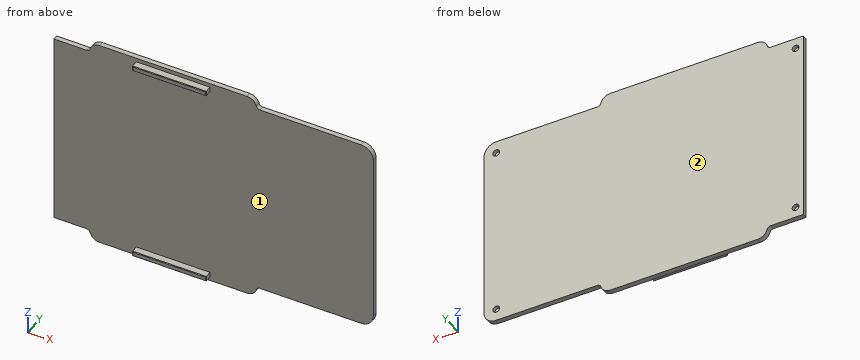
```python
from build123d import *

# Parameters (mm, degrees)
BOSS_EXTRUDE1_DEPTH = 4
FILLET1_R           = 3
FILLET2_R           = 8
FILLET3_R           = 10
SKETCH2_R           = 2.75
CUT_EXTRUDE2_DEPTH  = 4
SKETCH3_W           = 60
SKETCH3_H           = 4
BOSS_EXTRUDE2_DEPTH = 6
CHAMFER1_SIZE       = 0.5
SKETCH2_3_R         = 2.75
BOSS_EXTRUDE3_DEPTH = 1


with BuildPart() as part:
    # Sketch1 → Boss-Extrude1 (new body)
    with BuildSketch(Plane(origin=(0, 0, 0), x_dir=(1, 0, 0), z_dir=(0, 1, 0))):
        Polygon((29.5, 168.2), (29.5, 160), (0, 160), (0, 80), (0, 0), (29.5, 0), (29.5, -8.2), (164.72, -8.2), (164.72, 0), (260, 0), (260, 160), (164.72, 160), (164.72, 168.2), align=None)
    extrude(amount=BOSS_EXTRUDE1_DEPTH)

    # Fillet1
    fillet1_edges = [part.edges().sort_by_distance(p)[0] for p in [
        (164.72, 2, 0),
        (29.5, 2, 0),
        (29.5, 2, -160),
        (164.72, 2, -160),
    ]]
    fillet(fillet1_edges, radius=FILLET1_R)

    # Fillet2
    fillet2_edges = [part.edges().sort_by_distance(p)[0] for p in [
        (29.5, 2, -168.2),
        (164.72, 2, -168.2),
        (29.5, 2, 8.2),
        (164.72, 2, 8.2),
    ]]
    fillet(fillet2_edges, radius=FILLET2_R)

    # Fillet3
    fillet3_edges = [part.edges().sort_by_distance(p)[0] for p in [
        (260, 2, -160),
        (260, 2, 0),
    ]]
    fillet(fillet3_edges, radius=FILLET3_R)

    # Sketch2 → Cut-Extrude2 (cut)
    with BuildSketch(Plane(origin=(0, 0, 0), x_dir=(1, 0, 0), z_dir=(0, 1, 0))):
        with Locations((6.25, 151.25)):
            Circle(SKETCH2_R)
        with Locations((250, 150)):
            Circle(SKETCH2_R)
        with Locations((250, 10)):
            Circle(SKETCH2_R)
        with Locations((6.25, 8.75)):
            Circle(SKETCH2_R)
    extrude(amount=CUT_EXTRUDE2_DEPTH, mode=Mode.SUBTRACT)

    # Sketch3 → Boss-Extrude2 (add)
    with BuildSketch(Plane(origin=(0, 0, 0), x_dir=(1, 0, 0), z_dir=(0, 1, 0))):
        with Locations((97.11, 163)):
            Rectangle(SKETCH3_W, SKETCH3_H)
        with Locations((97.11, -3)):
            Rectangle(SKETCH3_W, SKETCH3_H)
    extrude(amount=-BOSS_EXTRUDE2_DEPTH)

    # Chamfer1
    chamfer1_edges = [part.edges().sort_by_distance(p)[0] for p in [
        (67.11, -6, -163),
        (97.11, -6, -161),
        (97.11, -6, -165),
        (127.11, -6, -163),
        (127.11, -6, 3),
        (97.11, -6, 5),
        (67.11, -6, 3),
        (97.11, -6, 1),
    ]]
    chamfer(chamfer1_edges, length=CHAMFER1_SIZE)

    # Sketch2<3> → Boss-Extrude3 (add)
    with BuildSketch(Plane(origin=(0, 0, 0), x_dir=(1, 0, 0), z_dir=(0, 1, 0))):
        with Locations((6.25, 151.25)):
            Circle(SKETCH2_3_R)
        with Locations((250, 150)):
            Circle(SKETCH2_3_R)
        with Locations((250, 10)):
            Circle(SKETCH2_3_R)
        with Locations((6.25, 8.75)):
            Circle(SKETCH2_3_R)
    extrude(amount=BOSS_EXTRUDE3_DEPTH)


solid = part.part
```
Design review of the part built by this model. Coordinates are the model's own, in mm. Face numbers are marked on the shaded views. Round coordinates to 2 decimals unless told otherwise and drop trailing zeros. Order: outer loops, then holes, each group sorted by start corner. A loop starts at its lowest first (then second) coordinate and runs counter-clockwise, first axis right, second up. Notation, with made-up numbers: (25, 19) - (55, 19) arc R30 ccw to (55, 44) - close; hole circle Ø8 at (53.25, 34). An arc over 180 degrees is marked (long way). Return JSON: item names as keys, results as strings.
Q1. Consider section C-C on z = -32. Write out the cut boundary in (x, y).
Computed values:
{"outline": "(0, 0) - (260, 0) - (260, 4) - (0, 4) - close"}
Q2. Consider section D-D on x = 122. Write out the cut boundary in (y, z), plus the area to 3 significant figures.
Computed values:
{"outline": "(-6, -164.5) - (-5.5, -165) - (0, -165) - (0, -168.2) - (4, -168.2) - (4, 8.2) - (0, 8.2) - (0, 5) - (-5.5, 5) - (-6, 4.5) - (-6, 1.5) - (-5.5, 1) - (0, 1) - (0, -161) - (-5.5, -161) - (-6, -161.5) - close", "area": "753 mm2"}
Q3. The part is to be moulded in two halves that separate along Z. For the marked faces 1 and 2, say which applies: pulls with the +Z half, pulls with the -Z half, needs draft (parallel to the pull), parting line crosses it, or undercut.
Computed values:
{"face 1": "undercut", "face 2": "needs draft"}
Q4. For pin 1 Ø3 at (x, y) = (228, 1.5) entering from +Z; pin 2 Ø3.5 at (x, z) = (6.25, -151.25) entering from -Y; pin 3 Ø1.2 at (x, y) = (14.5, 2) entering from -Z, all flat-tipped, find the tip position at first contact; note any pin that passes through.
Computed values:
{"pin 1": "stops at z = 0", "pin 2": "stops at y = 0", "pin 3": "stops at z = -160"}
Q5. Consider section B-B on x = 6.25. Write out the cut boundary in (y, z).
Computed values:
{"outline": "(0, -160) - (4, -160) - (4, -154) - (1, -154) - (1, -148.5) - (4, -148.5) - (4, -11.5) - (1, -11.5) - (1, -6) - (4, -6) - (4, 0) - (0, 0) - close"}
Q6. Consider section A-A on y = -2. Write out the cut boundary in (x, z).
Computed values:
{"outline": "(67.11, -165) - (127.11, -165) - (127.11, -161) - (67.11, -161) - close; (67.11, 1) - (127.11, 1) - (127.11, 5) - (67.11, 5) - close"}
Q7. Wall thickness on L1, parallel to Z at x = 250, y = 2.9; L2, parallel to Z at x = 6.25, y = 2.75; L3, parallel to X at y = 2.6, z = -8.75: over which ranges is each line inside the solid? List them lowest first. Write a range as [from, to].
Computed values:
{"L1": "z = [-160, -152.75], [-147.25, -12.75], [-7.25, 0]", "L2": "z = [-160, -154], [-148.5, -11.5], [-6, 0]", "L3": "x = [0, 3.5], [9, 247.55], [252.45, 259.92]"}
